Answer from the drawing. Dimensions are ordinates in mm from the lowest x, y and z of the part. A direction names the side the tool comes from. Coordinates: 2 decimals unless noted, no trailing zeros. Write each loop counter-clockwise with the first axis right and the second up, starting at its lowest first coordinate (ties: lowest second). Pieces come first, ordered by that corner, then holes. Notation, with made-up numbers: (44, 89.25) - (81, 89.25) arc R34 cw to (81, 127.25) - close; hole circle Ø1 at (18.5, -4). An arc over 180 degrees is marked (long way). Answer as a JSON object with one key per item and string values. Group by question number.
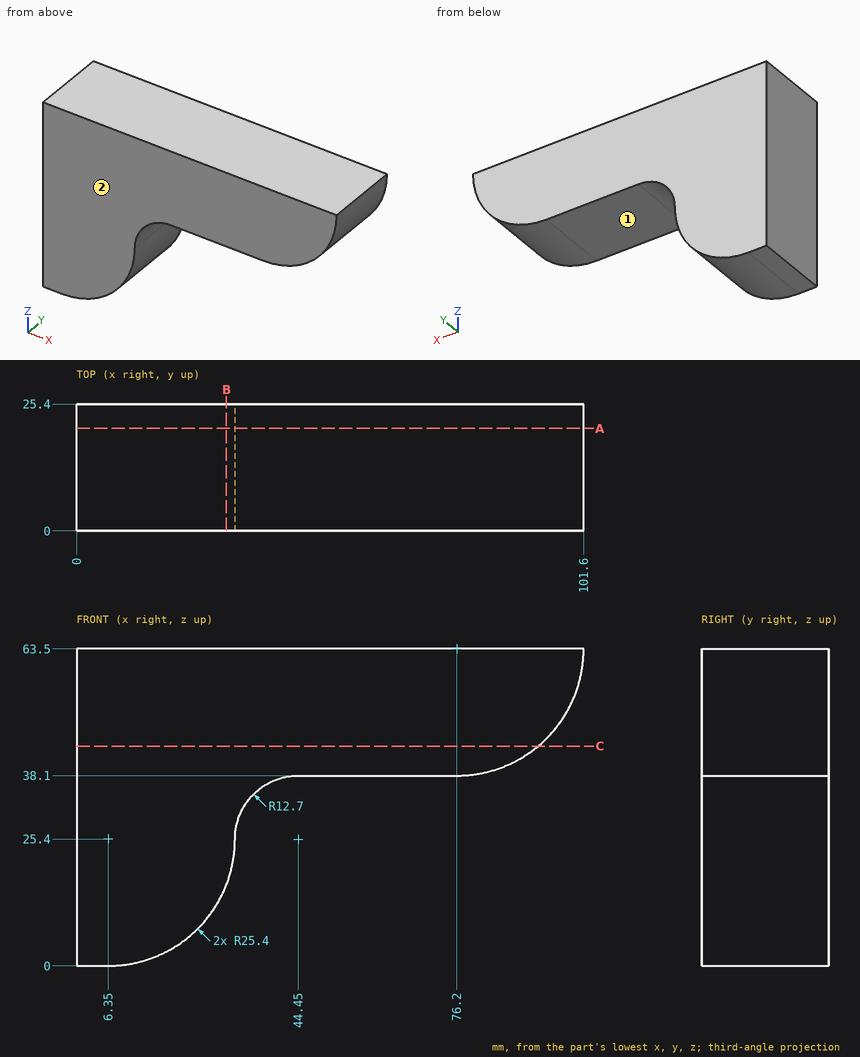
Q1. Section C-C on z = 44 is taken. Determine the outline of the cut face in (x, y), plus the area to 3 significant figures.
Q2. Section B-B on x = 30 is taken. Determine the outline of the cut face in (y, z).
Q3. Section A-A on y = 20.5 is taken. Determine the outline of the cut face in (x, z), plus the area to 3 significant figures.
Q4. Flat-ended cylindrical pins translate along their axes: pin 1 Ø2 at (x, y) = (90, 13) entering from -Z; pin 2 Ø5 at (x, z) = (51.5, 38) entering from +Y; pin 3 Ø12 at (x, y) = (16, 14.5) entering from -Z; pin 4 Ø12.5 at (x, y) = (65.5, 14) entering from -Z. Find the tip coordinate at first contact, or state that the pin passes through.
Q5. Consider L1, parallel to Z at x = 61, y = 23.5; L2, parallel to X at y = 17.25, z = 26; L3, parallel to Z at x = 88, y = 11.25. Determine where each line is inside the solid, lowest interval first. Write a range as from..to.
Q6. A tool of negligible diameter and unlimited length cuts with its end or side. For the marked faces 1 and 2, from which of +Z, -Z, +X, -X, +Y, -Y can it reach the whole face along a straight path? Write none if from no direction.
Numbers:
{
 "1": {"outline": "(0, 0) - (92.48, 0) - (92.48, 25.4) - (0, 25.4) - close", "area": "2,350 mm²"},
 "2": {"outline": "(0, 16.14) - (25.4, 16.14) - (25.4, 63.5) - (0, 63.5) - close"},
 "3": {"outline": "(0, 0) - (6.35, 0) arc R25.4 ccw to (31.75, 25.4) arc R12.7 cw to (44.45, 38.1) - (76.2, 38.1) arc R25.4 ccw to (101.6, 63.5) - (0, 63.5) - close", "area": "3,550 mm²"},
 "4": {"pin 1": "stops at z = 41.56", "pin 2": "stops at y = 25.4", "pin 3": "stops at z = 0.26", "pin 4": "stops at z = 38.1"},
 "5": {"L1": "z = 38.1..63.5", "L2": "x = 0..31.76", "L3": "z = 41.01..63.5"},
 "6": {"face 1": "-Z, +X, +Y, -Y", "face 2": "+Z, -Z, +X, -X, -Y"}
}
